Model file for the job. Use its own axes, mm. A direction names the side the tool comes from. Round coordinates to 2 decimals unless told otherwise and drop trailing zeros. Loops run counter-clockwise (first coordinate to the right, second up) from the corner with the lowest first, then second, coordinate; pieces in that order, holes last. Notation, with made-up numbers: M 30.25,10 L 45.25,10 A13 cw 45.25,17 Z; hole C -8,44 d1. An arc over 180 degrees is marked long. Use a Markdown table: item, result. Add a question column.
Item 1: Two-plate mould, pull along X, no slides. Class faces 1 (the flat face through (-16, -18.6, 3)), 2 (the flat face through (22.5, -29, 2)), 3 (the flat face through (17.5, 19, 3)), 4 (the flat face through (20, -20.1, 3)): +X half, -X half, draft (parallel to the pull), parting line (faces both ways), or undercut.
Item 2: Saw through at C-C on x = -9. Write the cut outline in (y, z), then the cut area to 3 significant figures.
Item 3: Pin check, flat tips, straight feed: P1, Ø1.7, axis at x = 16.5, z = 3, coming from the -Y side; P2, Ø2, axis at y = -15, z = 4, coming from the -X side; P3, Ø1.7, axis at x = 16, z = 3.5, coming from the +Y side. Stop position of each tip, or through.
Item 4: Saw through at D-D on y = -27. Write the cut outline in (x, z).
Item 5: Saw through at B-B on x = 11.5. Write the cut outline in (y, z), then the cut area to 3 significant figures.
Item 6: Wall check: L1, parallel to Y at x = 9, z = 0.55; L2, parallel to Y at x = 16, z = 1.55; L3, parallel to Y at x = 0, z = 1.95. Give the ranges that are in metal, low to high. Write a range as from..to.
Item 7: Tool access for faces 5 (the flat face through (-13, -32.5, 2)), 6 (the flat face through (16, 26, 3)), 7 (the flat face through (13, -32.5, 2)), 8 (the flat face through (-15, 32.5, 2)): list every direction of +Z, -Z, +X, -X, +Y, -Y with a clear straight run to the whole face (end or side of a thin tool).
Item 8: Saw through at A-A on x = 0. Write the cut outline in (y, z).
```python
from build123d import *

# Parameters (mm, degrees)
BOSS_EXTRUDE1_DEPTH = 5
CUT_EXTRUDE1_DEPTH  = 5
SKETCH10_R          = 4
SKETCH10_R_2        = 2
BOSS_EXTRUDE3_DEPTH = 5
SKETCH11_R          = 2
CUT_EXTRUDE3_DEPTH  = 5


with BuildPart() as part:
    # Sketch1 → Boss-Extrude1 (new body)
    with BuildSketch(Plane.XY):
        Polygon((7.5, 32.5), (7.5, 37.5), (-7.5, 37.5), (-7.5, 32.5), (-22.5, 32.5), (-22.5, 10), (-27.5, 10), (-27.5, -10), (-22.5, -10), (-22.5, -32.5), (22.5, -32.5), (22.5, 32.5), align=None)
    extrude(amount=BOSS_EXTRUDE1_DEPTH)

    # Sketch3 → Cut-Extrude1 (cut)
    with BuildSketch(Plane.XY.offset(5)):
        Polygon((22.5, 24.5), (17.5, 24.5), (17.5, 26), (14.1, 26), (14.1, 24.5), (7.5, 24.5), (7.5, 20.1), (14.1, 20.1), (14.1, 18.6), (17.5, 18.6), (17.5, 20.1), (22.5, 20.1), align=None)
        Polygon((22.5, -24.5), (22.5, -20.1), (17.5, -20.1), (17.5, -18.6), (14.1, -18.6), (14.1, -20.1), (7.5, -20.1), (7.5, -24.5), (14.1, -24.5), (14.1, -26), (17.5, -26), (17.5, -24.5), align=None)
        Polygon((-22.5, -24.5), (-17.5, -24.5), (-17.5, -26), (-14.1, -26), (-14.1, -24.5), (-7.5, -24.5), (-7.5, -20.1), (-14.1, -20.1), (-14.1, -18.6), (-17.5, -18.6), (-17.5, -20.1), (-22.5, -20.1), align=None)
    extrude(amount=-CUT_EXTRUDE1_DEPTH, mode=Mode.SUBTRACT)

    # Sketch10 → Boss-Extrude3 (add)
    with BuildSketch(Plane.XY.offset(5)):
        with Locations((0, -32.5)):
            Circle(SKETCH10_R)
        with Locations((0, -32.5)):
            Circle(SKETCH10_R_2, mode=Mode.SUBTRACT)
    extrude(amount=-BOSS_EXTRUDE3_DEPTH)

    # Sketch11 → Cut-Extrude3 (cut)
    with BuildSketch(Plane.XY.offset(5)):
        with Locations((0, -32.5)):
            Circle(SKETCH11_R)
    extrude(amount=-CUT_EXTRUDE3_DEPTH, mode=Mode.SUBTRACT)


solid = part.part
```
Entries:
| question | item | result |
|---|---|---|
| 1 | face 1 | undercut |
| 1 | face 2 | +X half |
| 1 | face 3 | undercut |
| 1 | face 4 | draft |
| 2 | outline | M -32.5,0 L -24.5,0 L -24.5,5 L -32.5,5 Z; M -20.1,0 L 32.5,0 L 32.5,5 L -20.1,5 Z |
| 2 | area | 303 mm2 |
| 3 | P1 | y = -32.5 |
| 3 | P2 | x = -22.5 |
| 3 | P3 | y = 32.5 |
| 4 | outline | M -22.5,0 L 22.5,0 L 22.5,5 L -22.5,5 Z |
| 5 | outline | M -32.5,0 L -24.5,0 L -24.5,5 L -32.5,5 Z; M -20.1,0 L 20.1,0 L 20.1,5 L -20.1,5 Z; M 24.5,0 L 32.5,0 L 32.5,5 L 24.5,5 Z |
| 5 | area | 281 mm2 |
| 6 | L1 | -32.5..-24.5, -20.1..20.1, 24.5..32.5 |
| 6 | L2 | -32.5..-26, -18.6..18.6, 26..32.5 |
| 6 | L3 | -36.5..-34.5, -30.5..37.5 |
| 7 | face 5 | +Z, -Z, -X, -Y |
| 7 | face 6 | +Z, -Z |
| 7 | face 7 | +Z, -Z, +X, -Y |
| 7 | face 8 | +Z, -Z, -X, +Y |
| 8 | outline | M -36.5,0 L -34.5,0 L -34.5,5 L -36.5,5 Z; M -30.5,0 L 37.5,0 L 37.5,5 L -30.5,5 Z |
